from build123d import *

# Parameters (mm, degrees)
F0_W     = 32
F0_H     = 40
F1_DEPTH = 120
F2_W     = 31
F2_H     = 39
F3_DEPTH = 120
F4_R     = 5
F5_R     = 5
F6_R     = 5
F7_R     = 5


with BuildPart() as f1:
    # F0 (on Front) → F1 (new body)
    with BuildSketch(Plane.XZ):
        with Locations((-36.2070729025, 39.3427484608)):
            Rectangle(F0_W, F0_H)
    extrude(amount=F1_DEPTH)

    # F2 (on face) → F3 (cut)
    with BuildSketch(Plane.XZ.offset(120)):
        with Locations((-36.1735836864, 39.8427484608)):
            Rectangle(F2_W, F2_H)
    extrude(amount=-F3_DEPTH, mode=Mode.SUBTRACT)

    # F4
    f4_edges = [f1.edges().sort_by_distance(p)[0] for p in [
        (-20.440328, -120, 59.342748),
    ]]
    fillet(f4_edges, radius=F4_R)

    # F5
    f5_edges = [f1.edges().sort_by_distance(p)[0] for p in [
        (-51.940328, -120, 59.342748),
    ]]
    fillet(f5_edges, radius=F5_R)

    # F6
    f6_edges = [f1.edges().sort_by_distance(p)[0] for p in [
        (-20.440328, 0, 59.342748),
    ]]
    fillet(f6_edges, radius=F6_R)

    # F7
    f7_edges = [f1.edges().sort_by_distance(p)[0] for p in [
        (-51.940328, 0, 59.342748),
    ]]
    fillet(f7_edges, radius=F7_R)


solid = f1.part
Check sheet for the modelled part. Datum: model origin and axes. Units: mm. A direction names the side the tool comes from. Round coordinates to 2 decimals unless told otherwise and drop trailing zeros. Write each loop counter-clockwise with the first axis right and the second up, starting at its lowest first coordinate (ties: lowest second). Pieces come first, ordered by that corner, then holes. Notation, with made-up numbers: (-2, 40) - (36, 40) arc R25 ccw to (36, 66) - close; hole circle Ø8 at (-22.75, -32.75). An arc over 180 degrees is marked (long way). Return JSON: item names as keys, results as strings.
Q1. Depth check by flat-ended pin: P1, Ø4, axis at x = -33.5, y = -27, coming from the +Z side. Enter the tip coordinate at first touch or a pass-through.
Returned:
{"P1": "stops at z = 20.34"}
Q2. Cross-section at A-A (z = 43.5). Record the boundary of the cut face in (x, y), then the cut area to 3 significant figures.
Returned:
{"outline": "(-52.21, -120) - (-51.67, -120) - (-51.67, 0) - (-52.21, 0) - close; (-20.67, -120) - (-20.21, -120) - (-20.21, 0) - (-20.67, 0) - close", "area": "120 mm²"}
Q3. Scan lines: L1, parallel to X at y = -100.5, z = 37; L2, parallel to Z at x = -23.5, y = -91. Record each from-to range of solid material in increasing order. Write a range as from..to.
Returned:
{"L1": "x = -52.21..-51.67, -20.67..-20.21", "L2": "z = 19.34..20.34"}
Q4. Cross-section at B-B (y = -100). Record the boundary of the cut face in (x, z).
Returned:
{"outline": "(-52.21, 19.34) - (-20.21, 19.34) - (-20.21, 59.34) - (-20.67, 59.34) - (-20.67, 20.34) - (-51.67, 20.34) - (-51.67, 59.34) - (-52.21, 59.34) - close"}
Q5. Access from +Z, -Z, +X, -X, +Y, -Y to the whole of each face (thin tool, end or side, straight path). Record for faces 4 (the cylindrical face through (-20.437, -1.426, 57.839)), 5 (the flat face through (-36, -61, 20.343)).
Returned:
{"face 4": "+Z, +X, -X, +Y", "face 5": "+Z, +Y, -Y"}
Q6. Draft check along X on faces 1 (the flat face through (-20.674, -61, 40)), 2 (the cylindrical face through (-20.437, -118.574, 57.839)), 3 (the flat face through (-52.207, -59, 39)). Enter one of: released by +X, released by -X, zero draft, split by the parting line, or undercut.
Returned:
{"face 1": "undercut", "face 2": "zero draft", "face 3": "released by -X"}
Q7. Cross-section at C-C (x = -25). Record the boundary of the cut face in (y, z), then the cut area to 3 significant figures.
Returned:
{"outline": "(-120, 19.34) - (0, 19.34) - (0, 20.34) - (-120, 20.34) - close", "area": "120 mm²"}
